Read the model definition and answer for the solid it produces. Units are mm, in the model's axes. Coordinates: 2 decimals unless noted, no trailing zeros. Write each loop counter-clockwise with the first axis right and the second up, starting at its lowest first coordinate (ties: lowest second). Pieces come first, ordered by that corner, then holes.
Item 1: Determine the mould class of faces 1 (the face through (0, 3, 5)), 2 (the face through (1.479, -5.538, 7.163)), 3 (the face through (3, 3, 5)) for opening direction X: released by +X, released by -X, zero draft, split by the parting line, or undercut.
Item 2: Section D-D (x = 2.65) is taken. Give the vertices of the cut face in (y, z), then the cut area to 3 significant figures.
Item 3: Section A-A (y = 0) is taken. Give the vertices of the cut face in (x, z).
Item 4: Each of these flat-tipped pins is pushed along its axis until it touches: P1, Ø1, axis at x = 2.5, y = -1, coming from the -Z side; P2, Ø2, axis at y = -6.32, z = -6.32, coming from the -X side; P3, Ø1.5, axis at x = 1.5, y = 6.5, coming from the -Z side. Where does it stop, or does it pass through?
Item 5: Section C-C (y = -6) is taken. Give the vertices of the cut face in (x, z), then the cut area to 3 significant figures.
Item 6: Straight lines are drawn through the part: probe 1 along Y at (x, z) = (1.1, 0); probe 2 along Y at (x, z) = (2.8, -5.75); probe 3 along Z at (x, y) = (2.6, 3.5). For each, find the intervals that lie inside material, in ascending order.
from build123d import *

# Parameters (mm, degrees)
SKETCH2_R           = 11
SKETCH2_R_2         = 5.6
BOSS_EXTRUDE1_DEPTH = 3
SKETCH3_R           = 1.15
CUT_EXTRUDE1_DEPTH  = 4


with BuildPart() as part:
    # Sketch2 → Boss-Extrude1 (new body)
    with BuildSketch(Plane(origin=(0, 0, 0), x_dir=(0, 0, -1), z_dir=(1, 0, 0))):
        Circle(SKETCH2_R)
        Circle(SKETCH2_R_2, mode=Mode.SUBTRACT)
    extrude(amount=BOSS_EXTRUDE1_DEPTH)

    # Sketch3 → Cut-Extrude1 (cut, through all)
    with BuildSketch(Plane(origin=(0, 0, 0), x_dir=(0, 0, -1), z_dir=(1, 0, 0))):
        with Locations((6.315465173, 6.315465173)):
            Circle(SKETCH3_R)
        with Locations((6.315465173, -6.315465173)):
            Circle(SKETCH3_R)
        with Locations((-6.315465173, -6.315465173)):
            Circle(SKETCH3_R)
        with Locations((-6.315465173, 6.315465173)):
            Circle(SKETCH3_R)
    extrude(amount=CUT_EXTRUDE1_DEPTH, mode=Mode.SUBTRACT)


solid = part.part
Established:
1. face 1: released by -X
1. face 2: zero draft
1. face 3: released by +X
2. outline: circle Ø22 at (0, 0); hole circle Ø2.3 at (-6.32, -6.32); hole circle Ø2.3 at (-6.32, 6.32); hole circle Ø11.2 at (0, 0); hole circle Ø2.3 at (6.32, -6.32); hole circle Ø2.3 at (6.32, 6.32)
2. area: 265 mm2
3. outline: (0, -11) - (3, -11) - (3, -5.6) - (0, -5.6) - close; (0, 5.6) - (3, 5.6) - (3, 11) - (0, 11) - close
4. P1: stops at z = -10.99
4. P2: passes through
4. P3: stops at z = -9.38
5. outline: (0, -9.22) - (3, -9.22) - (3, -7.42) - (0, -7.42) - close; (0, -5.21) - (3, -5.21) - (3, 5.21) - (0, 5.21) - close; (0, 7.42) - (3, 7.42) - (3, 9.22) - (0, 9.22) - close
5. area: 42.0 mm2
6. probe 1: y = -11 to -5.6, 5.6 to 11
6. probe 2: y = -9.38 to -7.32, -5.31 to 5.31, 7.32 to 9.38
6. probe 3: z = -10.43 to -4.37, 4.37 to 10.43
